from build123d import *

# Parameters (mm, degrees)
SKETCH1_R           = 10
BOSS_EXTRUDE1_DEPTH = 45
SCALE_1_SCALE       = 0.3
SKETCH_1_R          = 6
EXTRUDE_1_DEPTH     = 3
SKETCH_2_R          = 3
SKETCH_2_R_2        = 2.75
CUT_EXTRUDE_1_DEPTH = 13.5


with BuildPart() as part:
    # Sketch1 → Boss-Extrude1 (new body)
    with BuildSketch(Plane(origin=(0, 0, 0), x_dir=(1, 0, 0), z_dir=(0, 1, 0))):
        Circle(SKETCH1_R)
    extrude(amount=BOSS_EXTRUDE1_DEPTH)


with BuildPart() as part_1:
    # 축척1: scaled about (0, 22.5, 0)
    add(part.part.scale(SCALE_1_SCALE).moved(Location((0, 15.75, 0))))

    # 스케치1 → 보스-돌출1 (add)
    with BuildSketch(Plane(origin=(0, 29.25, 0), x_dir=(1, 0, 0), z_dir=(0, 1, 0))):
        Circle(SKETCH_1_R)
    extrude(amount=EXTRUDE_1_DEPTH)

    # 스케치2 → 컷-돌출1 (cut)
    with BuildSketch(Plane.XZ.offset(-15.75)):
        Circle(SKETCH_2_R)
        Circle(SKETCH_2_R_2, mode=Mode.SUBTRACT)
    extrude(amount=-CUT_EXTRUDE_1_DEPTH, mode=Mode.SUBTRACT)


solid = part_1.part
Read the model definition and answer for the solid it produces. Units are mm, in the model's axes. A direction names the side the tool comes from. Coordinates: 2 decimals unless noted, no trailing zeros. Order: outer loops, then holes, each group sorted by start corner. A loop starts at its lowest first (then second) coordinate and runs counter-clockwise, first axis right, second up. Notation, with made-up numbers: M -13.75,11 L 10.25,11 A19 cw 10.25,47 Z; hole C 79.5,-13.75 d10. An arc over 180 degrees is marked long. Put each result on its own line as item: value. Start each with the question number.
Item 1: Section B-B, the plane z = -1.5 is taken. Determine the outline of the cut face in (x, y), plus the area to 3 significant figures.
Item 2: Given pin 1 Ø1.5 at (x, y) = (4.5, 19) entering from +Z; pin 2 Ø1 at (y, z) = (19.5, 1) entering from -X, each flat-ended and moving along its own axis, determine where each tip first touches the part or whether it passes through.
Item 3: Section A-A, the plane x = 0 is taken. Determine the outline of the cut face in (y, z), plus the area to 3 significant figures.
Item 4: Section D-D, the plane y = 29.75 is taken. Determine the outline of the cut face in (x, z).
Item 5: Consider probe 1 along Y at (x, z) = (-3.5, 4.5); probe 2 along Z at (x, y) = (0, 21.75); probe 3 along X at (y, z) = (18.75, -0.5). Determine where each line is inside the solid, lowest interval first. Write a range as [from, to].
Item 6: Section C-C, the plane y = 27 is taken. Determine the outline of the cut face in (x, z).
Item 7: For faces 1 (the face through (3, 29.25, 1)), 2 (the face through (0, 15.75, 0)), determine the directions among +Z, -Z, +X, -X, +Y, -Y from which every point of the face is accessible in a straight line to the end or side of a thin tool.
Computed:
1. outline: M -5.81,29.25 L -2.3,29.25 L -2.3,15.75 L 2.3,15.75 L 2.3,29.25 L 5.81,29.25 L 5.81,32.25 L -5.81,32.25 Z
1. area: 97.1 mm2
2. pin 1: passes through
2. pin 2: stops at x = -2.7
3. outline: M 15.75,-2.75 L 29.25,-2.75 L 29.25,-6 L 32.25,-6 L 32.25,6 L 29.25,6 L 29.25,2.75 L 15.75,2.75 Z
3. area: 110 mm2
4. outline: C 0,0 d12
5. probe 1: y = [29.25, 32.25]
5. probe 2: z = [-2.75, 2.75]
5. probe 3: x = [-2.7, 2.7]
6. outline: C 0,0 d5.5
7. face 1: -Y
7. face 2: +Z, -Z, +X, -X, -Y
